```python
from build123d import *

# Parameters (mm, degrees)
SKETCH1_W           = 100
SKETCH1_H           = 100
BOSS_EXTRUDE1_DEPTH = 30
SKETCH2_R           = 44.45
SKETCH2_R_2         = 41.275
BOSS_EXTRUDE2_DEPTH = 2133.6


with BuildPart() as part:
    # Sketch1 → Boss-Extrude1 (new body, symmetric)
    with BuildSketch(Plane(origin=(0, 0, 0), x_dir=(1, 0, 0), z_dir=(0, 1, 0))):
        Rectangle(SKETCH1_W, SKETCH1_H)
    extrude(amount=BOSS_EXTRUDE1_DEPTH, both=True)

    # Sketch2 → Boss-Extrude2 (add)
    with BuildSketch(Plane(origin=(0, 30, 0), x_dir=(1, 0, 0), z_dir=(0, 1, 0))):
        Circle(SKETCH2_R)
        Circle(SKETCH2_R_2, mode=Mode.SUBTRACT)
    extrude(amount=BOSS_EXTRUDE2_DEPTH)


solid = part.part
```
Here's how the part is built. I have some questions about the finished solid (model axes, mm). A direction names the side the tool comes from. Give positions to 0.01 mm unless a question says otherwise; leave off trailing zeros. Write each loop counter-clockwise with the first axis right and the second up, starting at its lowest first coordinate (ties: lowest second). Pieces come first, ordered by that corner, then holes.
(1) On a 3-axis mill with a long thin cutter (end or side, diameter ignored), from which of +Z, -Z, +X, -X, +Y, -Y can I reach the whole of each face in a straight line? I mean faces 4 (the face through (-45, 30, -1)), 5 (the face through (-1, -30, -1)). Say none if no direction works.
Output values:
face 4: +Y
face 5: +Z, -Z, +X, -X, -Y
(2) Thinking about a two-plate mould opening in Z: for faces 1 (the face through (-1, 30, -1)), 2 (the face through (50, 0, 1)), 3 (the face through (-1, 0, 50)), which applies, pulls with the +Z half, pulls with the -Z half, needs draft (parallel to the pull), parting line crosses it, or undercut?
Output values:
face 1: undercut
face 2: needs draft
face 3: pulls with the +Z half
(3) Imagine slicing it at A-A, the plane z = 0. Write out the boundary of the cut face in (x, y) (3 decimals), and give its area (3 significant figures).
Output values:
outline: (-50, -30) - (50, -30) - (50, 30) - (44.45, 30) - (44.45, 2163.6) - (41.275, 2163.6) - (41.275, 30) - (-41.275, 30) - (-41.275, 2163.6) - (-44.45, 2163.6) - (-44.45, 30) - (-50, 30) - close
area: 19,500 mm2
(4) Imagine slicing it at B-B, the plane x = 0. Write out the boundary of the cut face in (y, z) (3 decimals).
Output values:
outline: (-30, -50) - (30, -50) - (30, -44.45) - (2163.6, -44.45) - (2163.6, -41.275) - (30, -41.275) - (30, 41.275) - (2163.6, 41.275) - (2163.6, 44.45) - (30, 44.45) - (30, 50) - (-30, 50) - close
(5) Imagine slicing it at C-C, the plane y = 1309. Write out the boundary of the cut face in (x, z) (3 decimals), and give its area (3 significant figures).
Output values:
outline: circle Ø88.9 at (0, 0); hole circle Ø82.55 at (0, 0)
area: 855 mm2
(6) If I drill on L1, parallel to X at y = 723, z = -2.5; L2, parallel to X at y = 880.5, z = 0 (3 decimals), over which ranges is the centre line in solid material (lowest first)?
Output values:
L1: x = -44.38 to -41.2, 41.2 to 44.38
L2: x = -44.45 to -41.275, 41.275 to 44.45
(7) Will these pins go through, and if not, where does the flat tip stop? pin 1 (10 mm diameter, centred on x = -10.5, y = 1367.5, fed in from -Z); pin 2 (5 mm diameter, centred on y = 452, z = -27.5, fed in from +X); pin 3 (10 mm diameter, centred on x = 10, y = 1655.5, fed in from +Z).
Output values:
pin 1: stops at z = -44.11
pin 2: stops at x = 36.75
pin 3: stops at z = 44.17
